from build123d import *

# Parameters (mm, degrees)
BOSS_EXTRUDE1_DEPTH = 3
SKETCH2_R           = 2.1
CUT_EXTRUDE1_DEPTH  = 4


with BuildPart() as part:
    # Sketch1 → Boss-Extrude1 (new body)
    with BuildSketch(Plane(origin=(0, 0, 0), x_dir=(1, 0, 0), z_dir=(0, 1, 0))):
        Polygon((15, 0), (20, 0), (20, -50), (23, -50), (23, -100), (20, -100), (20, -150), (0, -150), (0, -100), (-3, -100), (-3, -50), (0, -50), (0, 0), (5, 0), (5, 3), (15, 3), align=None)
    extrude(amount=BOSS_EXTRUDE1_DEPTH)

    # Sketch2 → Cut-Extrude1 (cut, through all)
    with BuildSketch(Plane(origin=(0, 3, 0), x_dir=(1, 0, 0), z_dir=(0, 1, 0))):
        with Locations((10, -35)):
            Circle(SKETCH2_R)
        with Locations((10, -50)):
            Circle(SKETCH2_R)
        with Locations((10, -83)):
            Circle(SKETCH2_R)
        with Locations((10, -133)):
            Circle(SKETCH2_R)
    extrude(amount=-CUT_EXTRUDE1_DEPTH, mode=Mode.SUBTRACT)


solid = part.part
Can you work these out from the model? Positions are in its coordinate system, mm. A direction names the side the tool comes from. Give positions to 0.01 mm unless a question says otherwise; leave off trailing zeros. Loops run counter-clockwise (first coordinate to the right, second up) from the corner with the lowest first, then second, coordinate; pieces in that order, holes last. Notation, with made-up numbers: (-3.75, 60) -> (37.25, 60) arc R30 ccw to (37.25, 96) -> close; hole circle Ø3 at (45, 40). An arc over 180 degrees is marked (long way). Write item = value, one per line.
1) Suppose I cut it at D-D on z = 83. Write out the boundary of the cut face in (x, y).
Check result:
outline = (-3, 0) -> (7.9, 0) -> (7.9, 3) -> (-3, 3) -> close; (12.1, 0) -> (23, 0) -> (23, 3) -> (12.1, 3) -> close
2) I need wall thicknesses on L1, parallel to Z at x = 10, y = 1.3; L2, parallel to X at y = 1.75, z = 35; L3, parallel to X at y = 2.4, z = 83. Which ranges of each line are inside material? Lowest first, please. Write a range as from..to.
Check result:
L1 = -3..32.9, 37.1..47.9, 52.1..80.9, 85.1..130.9, 135.1..150
L2 = 0..7.9, 12.1..20
L3 = -3..7.9, 12.1..23
3) Suppose I cut it at B-B on x = 10. Write out the boundary of the cut face in (y, z).
Check result:
outline = (0, -3) -> (3, -3) -> (3, 32.9) -> (0, 32.9) -> close; (0, 37.1) -> (3, 37.1) -> (3, 47.9) -> (0, 47.9) -> close; (0, 52.1) -> (3, 52.1) -> (3, 80.9) -> (0, 80.9) -> close; (0, 85.1) -> (3, 85.1) -> (3, 130.9) -> (0, 130.9) -> close; (0, 135.1) -> (3, 135.1) -> (3, 150) -> (0, 150) -> close
4) Thinking about a two-plate mould opening in X: for faces 1 (the cylindrical face through (8.334, 1.521, 36.278)), 2 (the flat face through (-2, 1, 50)), 3 (the flat face through (-3, 1, 75)), 4 (the cylindrical face through (8.334, 1.521, 84.278)), which applies, released by +X, released by -X, zero draft, split by the parting line, or undercut?
Check result:
face_1 = undercut
face_2 = zero draft
face_3 = released by -X
face_4 = undercut
5) For faces 5 (the flat face through (20, 1, 125)), 6 (the flat face through (-1, 1, 100)), 7 (the flat face through (17, 1, 0)), which set-ups out of +Z, -Z, +X, -X, +Y, -Y let a thin tool reach every point of the face, with its end or its side?
Check result:
face_5 = +Z, +X, +Y, -Y
face_6 = +Z, -X, +Y, -Y
face_7 = -Z, +X, +Y, -Y
6) Will these pins go through, and if not, where does the flat tip stop? pin 1 (1.5 mm diameter, centred on x = 2, y = 1.5, fed in from -Z); pin 2 (1.5 mm diameter, centred on y = 1, z = 131.5, fed in from -X); pin 3 (1.5 mm diameter, centred on y = 1, z = -2, fed in from -X); pin 4 (3.5 mm diameter, centred on x = 10, z = 50, fed in from +Y).
Check result:
pin_1 = 0
pin_2 = 0
pin_3 = 5
pin_4 = through
7) Suppose I cut it at C-C on y = 2.4. Write out the boundary of the cut face in (x, z).
Check result:
outline = (-3, 50) -> (0, 50) -> (0, 0) -> (5, 0) -> (5, -3) -> (15, -3) -> (15, 0) -> (20, 0) -> (20, 50) -> (23, 50) -> (23, 100) -> (20, 100) -> (20, 150) -> (0, 150) -> (0, 100) -> (-3, 100) -> close; hole circle Ø4.2 at (10, 35); hole circle Ø4.2 at (10, 50); hole circle Ø4.2 at (10, 83); hole circle Ø4.2 at (10, 133)
8) Suppose I cut it at A-A on z = 133. Write out the boundary of the cut face in (x, y).
Check result:
outline = (0, 0) -> (7.9, 0) -> (7.9, 3) -> (0, 3) -> close; (12.1, 0) -> (20, 0) -> (20, 3) -> (12.1, 3) -> close
